```python
from build123d import *

# Parameters (mm, degrees)
CROQUIS2_R              = 25
SALIENTE_EXTRUIR1_DEPTH = 100
CORTAR_EXTRUIR1_DEPTH   = 100
CROQUIS4_R              = 25
CORTAR_EXTRUIR2_DEPTH   = 100
CROQUIS5_W              = 40
CROQUIS5_H              = 50
CORTAR_EXTRUIR3_DEPTH   = 101


with BuildPart() as part:
    # Croquis2 → Saliente-Extruir1 (new body)
    with BuildSketch(Plane.XY):
        with BuildLine():
            Line((0, 0), (40, 0))
            Line((40, 0), (40, 150))
            Line((40, 150), (70, 150))
            Line((70, 150), (70, 250))
            ThreePointArc((70, 250), (20, 300), (-30, 250))
            Line((-30, 250), (-30, 150))
            Line((-30, 150), (0, 150))
            Line((0, 150), (0, 0))
        make_face()
        with Locations((20, 250)):
            Circle(CROQUIS2_R, mode=Mode.SUBTRACT)
    extrude(amount=SALIENTE_EXTRUIR1_DEPTH)

    # Croquis3 → Cortar-Extruir1 (cut)
    with BuildSketch(Plane(origin=(40, 0, 0), x_dir=(0, 0, -1), z_dir=(1, 0, 0))):
        with BuildLine():
            ThreePointArc((-50, 0), (-85.355339059, 14.644660941), (-100, 50))
            Line((-100, 50), (-100, 0))
            Line((-100, 0), (-50, 0))
        make_face()
        with BuildLine():
            ThreePointArc((0, 50), (-14.644660941, 14.644660941), (-50, 0))
            Line((-50, 0), (0, 0))
            Line((0, 0), (0, 50))
        make_face()
    extrude(amount=-CORTAR_EXTRUIR1_DEPTH, mode=Mode.SUBTRACT)

    # Croquis4 → Cortar-Extruir2 (cut)
    with BuildSketch(Plane(origin=(40, 0, 0), x_dir=(0, 0, -1), z_dir=(1, 0, 0))):
        with Locations((-50, 50)):
            Circle(CROQUIS4_R)
    extrude(amount=-CORTAR_EXTRUIR2_DEPTH, mode=Mode.SUBTRACT)

    # Croquis5 → Cortar-Extruir3 (cut, through all)
    with BuildSketch(Plane(origin=(70, 0, 0), x_dir=(0, 0, -1), z_dir=(1, 0, 0))):
        with Locations((-50, 275)):
            Rectangle(CROQUIS5_W, CROQUIS5_H)
        with Locations((-50, 225)):
            Rectangle(CROQUIS5_W, CROQUIS5_H)
    extrude(amount=-CORTAR_EXTRUIR3_DEPTH, mode=Mode.SUBTRACT)


solid = part.part
```
Source: CAD feature listing. Evaluate the final solid. Frame: model axes, mm. A direction names the side the tool comes from. Give positions to 0.01 mm unless a question says otherwise; leave off trailing zeros. Write each loop counter-clockwise with the first axis right and the second up, starting at its lowest first coordinate (ties: lowest second). Pieces come first, ordered by that corner, then holes.
1. Section query C-C (x = 5). Return the cut outline in (y, z).
2. Material intervals for line 1 along Y through (x, z) = (16.5, 50); line 2 along X through (y, z) = (250, 19.75); line 3 along Z through (x, y) = (-4, 219), sorted ascending.
3. Section query A-A (x = 20). Return the cut outline in (y, z), then the cut area to 3 significant figures.
4. Pull-direction query (X, two-part tool) for faces 1 (the face through (0, 93, 49)), 2 (the face through (20, 35, 70)), 3 (the face through (16.745, 274.787, 84.79)); classes: +X half, -X half, draft (parallel to the pull), parting line (faces both ways), or undercut.
5. Section query B-B (z = 57.5). Return the cut outline in (x, y), then the cut area to 3 significant figures.
6. First-contact query: pin 1 (6 mm diameter, centred on x = -12.5, z = 60, fed in from -Y); pin 2 (2 mm diameter, centred on x = 34.5, y = 40.5, fed in from +Z); pin 3 (5 mm diameter, centred on y = 50.5, z = 24, fed in from -X). Flat tips, straight axial feed; report the tip coordinate or a pass-through.
7. Access query for faces 4 (the face through (-15, 150, 49)), 5 (the face through (42.9, 239.6, 70)), 6 (the face through (40, 91, 49)). Directions: +Z, -Z, +X, -X, +Y, -Y. A direction counts if a zero-diameter tool reaches every point of the face in a straight line with its end or side. Return the directions, or none.
8. Section query D-D (z = 83). Return the cut outline in (x, y).
Output values:
1. outline: (50, 0) - (230, 0) - (230, 30) - (200, 30) - (200, 70) - (230, 70) - (230, 100) - (50, 100) arc R50 ccw to start; (270, 0) - (297.7, 0) - (297.7, 30) - (270, 30) - close; (270, 70) - (297.7, 70) - (297.7, 100) - (270, 100) - close; hole circle Ø50 at (50, 50)
2. line 1: y = 0 to 25, 75 to 200
2. line 2: x = -30 to -5, 45 to 70
2. line 3: z = 0 to 30, 70 to 100
3. outline: (50, 0) - (225, 0) - (225, 30) - (200, 30) - (200, 70) - (225, 70) - (225, 100) - (50, 100) arc R50 ccw to start; (275, 0) - (300, 0) - (300, 30) - (275, 30) - close; (275, 70) - (300, 70) - (300, 100) - (275, 100) - close; hole circle Ø50 at (50, 50)
3. area: 20,000 mm2
4. face 1: -X half
4. face 2: draft
4. face 3: undercut
5. outline: (-30, 150) - (0, 150) - (0, 73.85) - (40, 73.85) - (40, 150) - (70, 150) - (70, 200) - (-30, 200) - close; (0, 0.57) - (40, 0.57) - (40, 26.15) - (0, 26.15) - close
5. area: 9,070 mm2
6. pin 1: stops at y = 150
6. pin 2: stops at z = 99.27
6. pin 3: stops at x = 0
7. face 4: +Z, -Z, -X, -Y
7. face 5: +X, -X, +Y
7. face 6: +Z, -Z, +X, -Y
8. outline: (-30, 150) - (0, 150) - (0, 12.44) - (40, 12.44) - (40, 150) - (70, 150) - (70, 250) arc R50 ccw to (-30, 250) - close; hole circle Ø50 at (20, 250)
